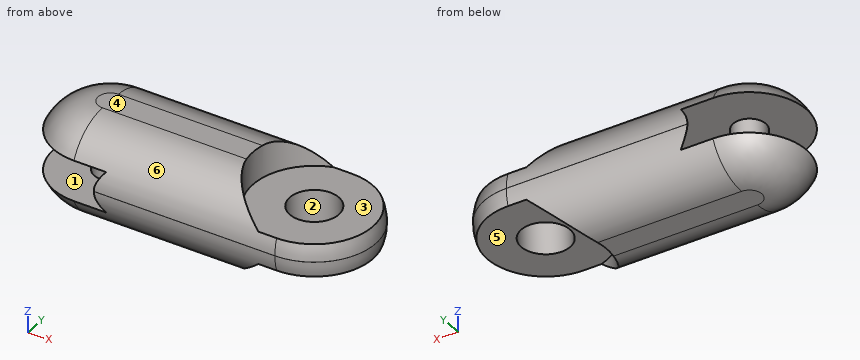
from build123d import *

# Parameters (mm, degrees)
PAD_DEPTH       = 6
FILLET_R        = 5.99
SKETCH001_R     = 8
POCKET_DEPTH    = 2.5
SKETCH002_R     = 7.5
POCKET001_DEPTH = 4.001
SKETCH003_R     = 7.5
POCKET002_DEPTH = 4.001
SKETCH004_R     = 3
POCKET003_DEPTH = 4
SKETCH005_R     = 2
PAD001_DEPTH    = 5


with BuildPart() as part:
    # Sketch → Pad (new body, symmetric)
    with BuildSketch(Plane.XY):
        with BuildLine():
            ThreePointArc((0, 7.5), (-7.5, 0), (0, -7.5))
            Line((0, -7.5), (25, -7.5))
            ThreePointArc((25, -7.5), (32.5, 0), (25, 7.5))
            Line((25, 7.5), (0, 7.5))
        make_face()
    extrude(amount=PAD_DEPTH, both=True)

    # Fillet
    fillet_edges = [part.edges().sort_by_distance(p)[0] for p in [
        (0, -7.5, 0),
        (25, -7.5, 0),
        (12.5, -7.5, -6),
        (12.5, -7.5, 6),
    ]]
    fillet(fillet_edges, radius=FILLET_R)

    # Sketch001 → Pocket (cut, symmetric)
    with BuildSketch(Plane.XY):
        Circle(SKETCH001_R)
    extrude(amount=POCKET_DEPTH, both=True, mode=Mode.SUBTRACT)

    # Sketch002 → Pocket001 (cut, through all)
    with BuildSketch(Plane.XY.offset(2)):
        with Locations((25, 0)):
            Circle(SKETCH002_R)
    extrude(amount=POCKET001_DEPTH, mode=Mode.SUBTRACT)

    # Sketch003 → Pocket002 (cut, through all)
    with BuildSketch(Plane.XY.offset(-2)):
        with Locations((25, 0)):
            Circle(SKETCH003_R)
    extrude(amount=-POCKET002_DEPTH, mode=Mode.SUBTRACT)

    # Sketch004 (on Face17 of Pocket002) → Pocket003 (cut)
    with BuildSketch(Plane.XY.offset(2)):
        with Locations((25, 0)):
            Circle(SKETCH004_R)
    extrude(amount=-POCKET003_DEPTH, mode=Mode.SUBTRACT)

    # Sketch005 (on Face6 of Pocket003) → Pad001 (join)
    with BuildSketch(Plane.XY.offset(-2.5)):
        Circle(SKETCH005_R)
    extrude(amount=PAD001_DEPTH)


solid = part.part
Design review of the part built by this model. Coordinates are the model's own, in mm. Face numbers are marked on the shaded views. A direction names the side the tool comes from. Give positions to 0.01 mm unless a question says otherwise; leave off trailing zeros. Use CSV: the item, a comma, the result in double quotes. Start each with the question number.
1. Wall thickness on L1, parallel to Z at x = 3.5, y = -1.25; L2, parallel to Y at x = 25, z = -0.1; L3, parallel to Z at x = -1, y = -1.25: over which ranges is each line inside the solid? List them lowest first.
2. Add section A-A (y = 0). Count the separate pieces of the cut face and the enclosed holes in it, plus the area to 3 significant figures.
3. Draft analysis for pull direction Y (two halves, no side actions). For the marked faces 4, 5 and 6, state which applies: released by +Y, released by -Y, zero draft, split by the parting line, or undercut.
4. Insertion check: P1, Ø7, axis at x = 23, y = -2, coming from the +Z side; P2, Ø1.5, axis at y = -4, z = -3, coming from the -X side; P3, Ø1.5, axis at y = -0.5, z = -2.5, coming from the +X side. Each pin has a flat end and moves straight along its axis. Give the tip position at first contact, or say it passes through.
5. Machinability: for the marked faces 1, 2 and 3, which of the approach directions +Z, -Z, +X, -X, +Y, -Y give a long, thin tool a straight path to every point of the face, cutting with its end or side? Answer none if there is none.
Results found:
1,L1,"z = -6 to -2.5, 2.5 to 6"
1,L2,"y = -7.5 to -3, 3 to 7.5"
1,L3,"z = -6 to 6"
2,separate pieces,"2"
2,enclosed holes,"1"
2,area,"264 mm²"
3,face 4,"zero draft"
3,face 5,"undercut"
3,face 6,"released by -Y"
4,P1,"stops at z = 2"
4,P2,"stops at x = -6.05"
4,P3,"stops at x = 32.23"
5,face 1,"none"
5,face 2,"+Z, -Z"
5,face 3,"+Z, +X"
